Answer from the drawing. Dimensions are ordinates in mm from the lowest x, y and z of the part. Coordinates: 2 decimals unless noted, no trailing zeros. Write each loop counter-clockwise with the first axis right and the second up, starting at its lowest first coordinate (ties: lowest second). Pieces come first, ordered by that corner, then holes. Notation, with made-up numbers: (26, 31.25) - (51, 31.25) arc R17 cw to (51, 48.25) - close; hole circle Ø4 at (55, 31). An arc over 180 degrees is marked (long way). Use one line per item in the form item = value. Start each with the question number.
Item 1: Consider probe 1 along X at (y, z) = (0.5, 5). Determine where the line is inside the solid, lowest interval first.
Item 2: A cutting plane is placed at B-B (z = 12.7). Write down the section's boundary in (x, y) (1 decimal).
Item 3: A cutting plane is placed at A-A (x = 44.45). Give the number of separate pieces and of enclosed holes in the cut face, then the cut area to 3 significant figures.
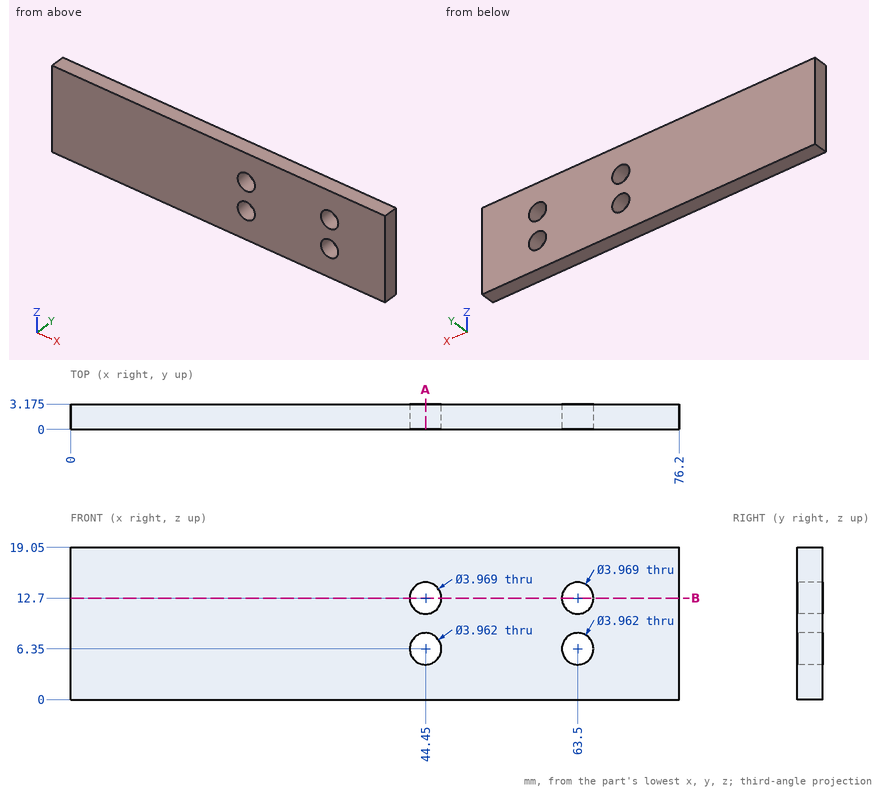
Answer:
q1.probe_1 = 0 to 43, 45.9 to 62.05, 64.95 to 76.2
q2.outline = (0, 0) - (42.5, 0) - (42.5, 3.2) - (0, 3.2) - close; (46.4, 0) - (61.5, 0) - (61.5, 3.2) - (46.4, 3.2) - close; (65.5, 0) - (76.2, 0) - (76.2, 3.2) - (65.5, 3.2) - close
q3.separate_pieces = 3
q3.enclosed_holes = 0
q3.area = 35.3 mm²
